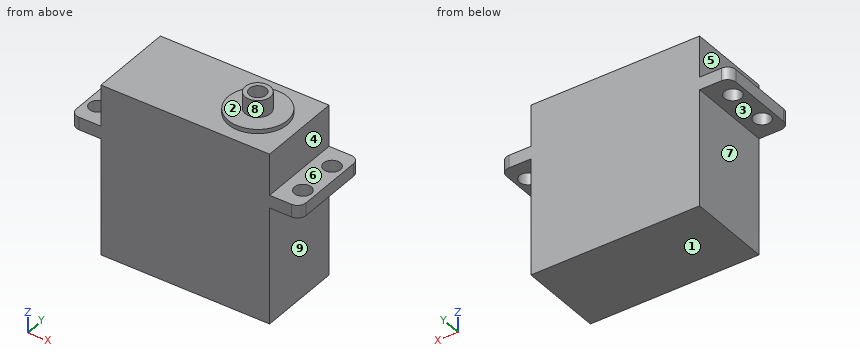
from build123d import *

# Parameters (mm, degrees)
SKETCH2_W           = 40
SKETCH2_H           = 20
BOSS_EXTRUDE1_DEPTH = 27.65
SKETCH3_W           = 54.44
SKETCH3_H           = 20
SKETCH3_R           = 2
BOSS_EXTRUDE2_DEPTH = 3
SKETCH4_W           = 40
SKETCH4_H           = 20
BOSS_EXTRUDE3_DEPTH = 9.8
SKETCH5_R           = 7
BOSS_EXTRUDE4_DEPTH = 1
SKETCH6_R           = 3
BOSS_EXTRUDE5_DEPTH = 4
FILLET1_R           = 2
SKETCH7_R           = 2
CUT_EXTRUDE1_DEPTH  = 10


with BuildPart() as part:
    # Sketch2 → Boss-Extrude1 (new body)
    with BuildSketch(Plane.XY):
        with Locations((-33.592215537, 218.387921433)):
            Rectangle(SKETCH2_W, SKETCH2_H)
    extrude(amount=BOSS_EXTRUDE1_DEPTH)

    # Sketch3 → Boss-Extrude2 (add)
    with BuildSketch(Plane.XY.offset(27.65)):
        with Locations((-33.592215537, 218.387921433)):
            Rectangle(SKETCH3_W, SKETCH3_H)
        with Locations((-9.292215537, 213.487921433)):
            Circle(SKETCH3_R, mode=Mode.SUBTRACT)
        with Locations((-9.292215537, 223.287921433)):
            Circle(SKETCH3_R, mode=Mode.SUBTRACT)
        with Locations((-57.892215537, 223.287921433)):
            Circle(SKETCH3_R, mode=Mode.SUBTRACT)
        with Locations((-57.892215537, 213.487921433)):
            Circle(SKETCH3_R, mode=Mode.SUBTRACT)
    extrude(amount=BOSS_EXTRUDE2_DEPTH)

    # Sketch4 → Boss-Extrude3 (add)
    with BuildSketch(Plane.XY.offset(30.65)):
        with Locations((-33.592215537, 218.387921433)):
            Rectangle(SKETCH4_W, SKETCH4_H)
    extrude(amount=BOSS_EXTRUDE3_DEPTH)

    # Sketch5 → Boss-Extrude4 (add)
    with BuildSketch(Plane.XY.offset(40.45)):
        with Locations((-23.442215537, 218.387921433)):
            Circle(SKETCH5_R)
    extrude(amount=BOSS_EXTRUDE4_DEPTH)

    # Sketch6 → Boss-Extrude5 (add)
    with BuildSketch(Plane.XY.offset(41.45)):
        with Locations((-23.442215537, 218.387921433)):
            Circle(SKETCH6_R)
    extrude(amount=BOSS_EXTRUDE5_DEPTH)

    # Fillet1
    fillet1_edges = [part.edges().sort_by_distance(p)[0] for p in [
        (-6.372215537, 208.387921433, 29.15),
        (-60.812215537, 208.387921433, 29.15),
        (-6.372215537, 228.387921433, 29.15),
        (-60.812215537, 228.387921433, 29.15),
    ]]
    fillet(fillet1_edges, radius=FILLET1_R)

    # Sketch7 → Cut-Extrude1 (cut)
    with BuildSketch(Plane.XY.offset(45.45)):
        with Locations((-23.442215537, 218.387921433)):
            Circle(SKETCH7_R)
    extrude(amount=-CUT_EXTRUDE1_DEPTH, mode=Mode.SUBTRACT)


solid = part.part
Can you work these out from the model? Positions are in its coordinate system, mm. Face numbers are marked on the shaded views. A direction names the side the tool comes from. Give positions to 0.01 mm unless a question says otherwise; leave off trailing zeros. Loops run counter-clockwise (first coordinate to the right, second up) from the corner with the lowest first, then second, coordinate; pieces in that order, holes last. Notation, with made-up numbers: (-4, 38) -> (27, 38) arc R21 cw to (27, 43) -> close; hole circle Ø2 at (72, 48). An arc over 180 degrees is marked (long way). Write item = value, one per line.
1) Thinking about a two-plate mould opening in X: for the marked faces 6, 7, 8 and 9, which applies, released by +X, released by -X, zero draft, split by the parting line, or undercut?
Check result:
face_6 = zero draft
face_7 = released by -X
face_8 = split by the parting line
face_9 = released by +X
2) Suppose I cut it at B-B on z = 38.5. Write out the boundary of the cut face in (x, y), then the cut area to 3 significant figures.
Check result:
outline = (-53.59, 208.39) -> (-13.59, 208.39) -> (-13.59, 228.39) -> (-53.59, 228.39) -> close; hole circle Ø4 at (-23.44, 218.39)
area = 787 mm2
3) Will these pins go through, and if not, where does the flat tip stop? pin 1 (6.5 mm diameter, centred on x = -9.29, y = 213.49, fed in from +Z); pin 2 (6 mm diameter, centred on x = -29.5, y = 213.5, fed in from +Z); pin 3 (2.5 mm diameter, centred on x = -57.89, y = 223.29, fed in from -Z); pin 4 (8 mm diameter, centred on x = -50.5, y = 215, fed in from +Z).
Check result:
pin_1 = 30.65
pin_2 = 41.45
pin_3 = through
pin_4 = 40.45
4) Suppose I cut it at C-C on y = 219.5. Write out the boundary of the cut face in (x, z).
Check result:
outline = (-60.81, 27.65) -> (-53.59, 27.65) -> (-53.59, 0) -> (-13.59, 0) -> (-13.59, 27.65) -> (-6.37, 27.65) -> (-6.37, 30.65) -> (-13.59, 30.65) -> (-13.59, 40.45) -> (-16.53, 40.45) -> (-16.53, 41.45) -> (-20.66, 41.45) -> (-20.66, 45.45) -> (-21.78, 45.45) -> (-21.78, 35.45) -> (-25.1, 35.45) -> (-25.1, 45.45) -> (-26.23, 45.45) -> (-26.23, 41.45) -> (-30.35, 41.45) -> (-30.35, 40.45) -> (-53.59, 40.45) -> (-53.59, 30.65) -> (-60.81, 30.65) -> close
5) Suppose I cut it at D-D on z = 11. Write out the boundary of the cut face in (x, y), then the cut area to 3 significant figures.
Check result:
outline = (-53.59, 208.39) -> (-13.59, 208.39) -> (-13.59, 228.39) -> (-53.59, 228.39) -> close
area = 800 mm2
6) Suppose I cut it at A-A on x = -9.5. Write out the boundary of the cut face in (y, z).
Check result:
outline = (208.39, 27.65) -> (211.5, 27.65) -> (211.5, 30.65) -> (208.39, 30.65) -> close; (215.48, 27.65) -> (221.3, 27.65) -> (221.3, 30.65) -> (215.48, 30.65) -> close; (225.28, 27.65) -> (228.39, 27.65) -> (228.39, 30.65) -> (225.28, 30.65) -> close
7) I need wall thicknesses on L1, parallel to Z at x = -32.5, y = 214.5; L2, parallel to X at y = 220, z = 9; L3, parallel to Z at x = -10, y = 209.75. Which ranges of each line are inside material? Lowest first, please. Write a range as from..to.
Check result:
L1 = 0..40.45
L2 = -53.59..-13.59
L3 = 27.65..30.65
8) For the marked faces 1, 2, 3, 4 and 5, which set-ups out of +Z, -Z, +X, -X, +Y, -Y let a thin tool reach every point of the face, with its end or its side?
Check result:
face_1 = -Z, +X, -X, +Y, -Y
face_2 = +Z
face_3 = -Z, -X, +Y, -Y
face_4 = +Z, +X, +Y, -Y
face_5 = +Z, -X, +Y, -Y
